from build123d import *
from build123d.topology import SkipClean

# Parameters (mm, degrees)
SKETCH1_W                      = 120
SKETCH1_H                      = 60
BOSS_EXTRUDE1_DEPTH            = 30
SKETCH2_R                      = 30
BOSS_EXTRUDE2_DEPTH            = 60
FILLET1_R                      = 15
SKETCH3_R                      = 5
CUT_EXTRUDE2_DEPTH             = 81.777472107
SKETCH4_R                      = 10
CUT_EXTRUDE3_DEPTH             = 22
CHAMFER1_SIZE                  = 1
SKETCH5_R                      = 15
CUT_EXTRUDE4_DEPTH             = 114.247516582
CHAMFER3_SIZE                  = 3
G1_16_TAPPED_HOLE2_D           = 6.6
G1_16_TAPPED_HOLE2_DEPTH       = 29.999
G1_16_TAPPED_HOLE2_CSINK_D     = 7.773
G1_16_TAPPED_HOLE2_CSINK_ANGLE = 90
G1_16_TAPPED_HOLE2_TIP         = 1.982840043


# Read off the part's stored shape, not the designer's step: Mirror1
with BuildPart() as part:
    # Sketch1 → Boss-Extrude1 (new body)
    with BuildSketch(Plane(origin=(0, 0, 0), x_dir=(1, 0, 0), z_dir=(0, 1, 0))):
        Rectangle(SKETCH1_W, SKETCH1_H)
    extrude(amount=BOSS_EXTRUDE1_DEPTH)

    # Sketch2 → Boss-Extrude2 (add)
    with BuildSketch(Plane.XY.offset(30)):
        with Locations((0, 45)):
            Circle(SKETCH2_R)
    extrude(amount=-BOSS_EXTRUDE2_DEPTH)

    # Fillet1
    fillet1_edges = [part.edges().sort_by_distance(p)[0] for p in [
        (-25.980762114, 30, 0),
    ]]
    fillet(fillet1_edges, radius=FILLET1_R)

    # Sketch3 → Cut-Extrude2 (cut, symmetric)
    with BuildSketch(Plane(origin=(0, 30, 0), x_dir=(1, 0, 0), z_dir=(0, 1, 0))):
        with Locations(Location((-45, 0, 0), (0, 0, 270))):
            Circle(SKETCH3_R)
    extrude(amount=CUT_EXTRUDE2_DEPTH, both=True, mode=Mode.SUBTRACT)

    # Sketch4 → Cut-Extrude3 (cut)
    with BuildSketch(Plane(origin=(0, 30, 0), x_dir=(1, 0, 0), z_dir=(0, 1, 0))):
        with Locations((-45, 0)):
            Circle(SKETCH4_R)
    extrude(amount=CUT_EXTRUDE3_DEPTH, mode=Mode.SUBTRACT)

    # Chamfer1
    chamfer1_edges = [part.edges().sort_by_distance(p)[0] for p in [
        (-45, 30, -5),
    ]]
    chamfer(chamfer1_edges, length=CHAMFER1_SIZE)

    # Sketch5 → Cut-Extrude4 (cut, through all)
    with BuildSketch(Plane.XY.offset(30)):
        with Locations((0, 45)):
            Circle(SKETCH5_R)
    extrude(amount=-CUT_EXTRUDE4_DEPTH, mode=Mode.SUBTRACT)

    # Chamfer3
    chamfer3_edges = [part.edges().sort_by_distance(p)[0] for p in [
        (-15, 45, -30),
        (-15, 45, 30),
    ]]
    chamfer(chamfer3_edges, length=CHAMFER3_SIZE)

    # Mirror1
    split(bisect_by=Plane(origin=(0, 0, 0), x_dir=(0, 0, 1), z_dir=(1, 0, 0)), keep=Keep.BOTTOM)

    # Mirror1 2: part across plane


with BuildPart() as part_1:
    with SkipClean():  # the faces are left unmerged after this step: merging them gives an invalid solid
        add(part.part)
        add(part.part.mirror(Plane(origin=(0, 0, 0), x_dir=(0, 0, 1), z_dir=(1, 0, 0))))

    # G1/16 Tapped Hole2
    with Locations(Plane(origin=(0, 75, 0), x_dir=(1, 0, 0), z_dir=(0, 1, 0))):
        with Locations((0, 0)):
            CounterSinkHole(G1_16_TAPPED_HOLE2_D / 2, G1_16_TAPPED_HOLE2_CSINK_D / 2, depth=G1_16_TAPPED_HOLE2_DEPTH, counter_sink_angle=G1_16_TAPPED_HOLE2_CSINK_ANGLE)
            with Locations((0, 0, -(G1_16_TAPPED_HOLE2_DEPTH + G1_16_TAPPED_HOLE2_TIP / 2))):  # 118° drill point
                Cone(0, G1_16_TAPPED_HOLE2_D / 2, G1_16_TAPPED_HOLE2_TIP, mode=Mode.SUBTRACT)


solid = part_1.part
CAD build for the part. Positions are in the model's coordinates, mm. A direction names the side the tool comes from. Round coordinates to 2 decimals unless told otherwise and drop trailing zeros. Loops run counter-clockwise (first coordinate to the right, second up) from the corner with the lowest first, then second, coordinate; pieces in that order, holes last.
(1) Drop flat-ended pins along their axis: pin 1 (16 mm diameter, centred on x = 45, z = 0, fed in from +Y); pin 2 (12.5 mm diameter, centred on x = -41.5, z = -2.5, fed in from +Y); pin 3 (1.5 mm diameter, centred on y = 50.5, z = 3, fed in from -X). Give the stop position or say it passes through.
(2) Wall check: line 1 along X through (y, z) = (19.25, 0); line 2 along Z through (x, y) = (0, 71); line 3 along X through (y, z) = (45.5, -10). Give the ranges that are in metal, low to high.
(3) Cut at A-A (z = 12). Give the cut face in (x, y), plus the area to 3 significant figures.
(4) Cut at B-B (y = 69). Give the cut face in (x, z).
(5) Cut at D-D (y = 23). Give the cut face in (x, z), plus the area to 3 significant figures.
(6) Which spindle directions (+Z, -Z, +X, -X, +Y, -Y) get a long thin tool onto all of the face, cutting with end or side? Do faces 1 (the cylindrical face through (35, 31, 0)), 2 (the cylindrical face through (-35, 31, 0)), 3 (the flat face through (-60, 15, 0)), 4 (the cylindrical face through (2.43, 66.92, -2.23)). Say none if no direction does.
(7) Cut at C-C (z = 0). Give the cut face in (x, y), plus the area to 3 significant figures.
Findings below:
1. pin 1: stops at y = 30
1. pin 2: stops at y = 33.6
1. pin 3: stops at x = -29.62
2. line 1: x = -60 to -50, -40 to 40, 50 to 60
2. line 2: z = -30 to -3.3, 3.3 to 30
2. line 3: x = -30 to -14.99, 14.99 to 30
3. outline: (-60, 0) - (60, 0) - (60, 30) - (45, 30) arc R15 cw to (30, 45) arc R30 ccw to (-30, 45) arc R15 cw to (-45, 30) - (-60, 30) - close; hole circle Ø30 at (0, 45)
3. area: 5,300 mm2
4. outline: (-18, -30) - (18, -30) - (18, 30) - (-18, 30) - close; hole circle Ø6.6 at (0, 0)
5. outline: (-60, -30) - (60, -30) - (60, 30) - (-60, 30) - close; hole circle Ø10 at (-45, 0); hole circle Ø10 at (45, 0)
5. area: 7,040 mm2
6. face 1: +X, +Y
6. face 2: -X, +Y
6. face 3: +Z, -Z, -X, +Y, -Y
6. face 4: +Y
7. outline: (-60, 0) - (-50, 0) - (-50, 29) - (-51, 30) - (-60, 30) - close; (-40, 0) - (40, 0) - (40, 29) - (39, 30) - (35, 30) - (35, 33.82) arc R15 cw to (30, 45) arc R30 ccw to (3.66, 74.78) - (3.3, 74.41) - (3.3, 59.63) arc R15 cw (long way) to (-3.3, 59.63) - (-3.3, 74.41) - (-3.66, 74.78) arc R30 ccw to (-30, 45) arc R15 cw to (-35, 33.82) - (-35, 30) - (-39, 30) - (-40, 29) - close; (50, 0) - (60, 0) - (60, 30) - (51, 30) - (50, 29) - close
7. area: 4,580 mm2
